```python
from build123d import *

# Parameters (mm, degrees)
SKETCH_R        = 11
PAD_DEPTH       = 15
SKETCH001_R     = 11
SKETCH001_R_2   = 5.1
POCKET_DEPTH    = 1.5
SKETCH002_R     = 11
SKETCH002_R_2   = 5.1
POCKET001_DEPTH = 10
SKETCH003_R     = 1.75
POCKET002_DEPTH = 13.501
SKETCH004_R     = 4
POCKET003_DEPTH = 15.001


with BuildPart() as part:
    # Sketch → Pad (new body)
    with BuildSketch(Plane.XY):
        Circle(SKETCH_R)
    extrude(amount=PAD_DEPTH)

    # Sketch001 (on Face3 of Pad) → Pocket (cut)
    with BuildSketch(Plane.XY.offset(15)):
        Circle(SKETCH001_R)
        Circle(SKETCH001_R_2, mode=Mode.SUBTRACT)
    extrude(amount=-POCKET_DEPTH, mode=Mode.SUBTRACT)

    # Sketch002 (on Face2 of Pocket) → Pocket001 (cut)
    with BuildSketch(Plane(origin=(0, 0, 0), x_dir=(1, 0, 0), z_dir=(0, 0, -1))):
        Circle(SKETCH002_R)
        Circle(SKETCH002_R_2, mode=Mode.SUBTRACT)
    extrude(amount=-POCKET001_DEPTH, mode=Mode.SUBTRACT)

    # Sketch003 (on Face3 of Pocket001) → Pocket002 (cut, through all)
    with BuildSketch(Plane.XY.offset(13.5)):
        with Locations((8, 0)):
            Circle(SKETCH003_R)
        with Locations((-8, 0)):
            Circle(SKETCH003_R)
        with Locations((0, 8)):
            Circle(SKETCH003_R)
        with Locations((0, -8)):
            Circle(SKETCH003_R)
    extrude(amount=-POCKET002_DEPTH, mode=Mode.SUBTRACT)

    # Sketch004 (on Face11 of Pocket002) → Pocket003 (cut, through all)
    with BuildSketch(Plane.XY.offset(15)):
        Circle(SKETCH004_R)
    extrude(amount=-POCKET003_DEPTH, mode=Mode.SUBTRACT)


solid = part.part
```
Here's how the part is built. I have some questions about the finished solid (model axes, mm). A direction names the side the tool comes from. Coordinates: 2 decimals unless noted, no trailing zeros. Loops run counter-clockwise (first coordinate to the right, second up) from the corner with the lowest first, then second, coordinate; pieces in that order, holes last. Notation, with made-up numbers: M 9,76.5 L 15,76.5 A17 cw 15,93.5 Z; hole C 7.5,-7.75 d6. An arc over 180 degrees is marked long. One line per item, written item: value.
1. Imagine slicing it at C-C (y = 0.5). List the corners of the cut face in (x, z) for me.
Geometry says:
outline: M -10.99,10 L -9.68,10 L -9.68,13.5 L -10.99,13.5 Z; M -6.32,10 L -5.08,10 L -5.08,0 L -3.97,0 L -3.97,15 L -5.08,15 L -5.08,13.5 L -6.32,13.5 Z; M 3.97,0 L 5.08,0 L 5.08,10 L 6.32,10 L 6.32,13.5 L 5.08,13.5 L 5.08,15 L 3.97,15 Z; M 9.68,10 L 10.99,10 L 10.99,13.5 L 9.68,13.5 Z
2. On a 3-axis mill with a long thin cutter (end or side, diameter ignored), from which of +Z, -Z, +X, -X, +Y, -Y can I reach the whole of each face in a straight line? I mean faces 1 (the cylindrical face through (2.4, -4.5, 14.3)), 2 (the flat face through (2, 5, 10)), 3 (the flat face through (-3, -3, 15)). Say none if no direction works.
Geometry says:
face 1: +Z
face 2: -Z
face 3: +Z, +X, -X, +Y, -Y
3. Imagine slicing it at D-D (z = 13). List the corners of the cut face in (x, y) for me.
Geometry says:
outline: C 0,0 d22; hole C -8,0 d3.5; hole C 0,0 d8; hole C 0,-8 d3.5; hole C 0,8 d3.5; hole C 8,0 d3.5
4. Imagine slicing it at B-B (x = -8). List the corners of the cut face in (y, z) for me, and give its area (3 significant figures).
Geometry says:
outline: M -7.55,10 L -1.75,10 L -1.75,13.5 L -7.55,13.5 Z; M 1.75,10 L 7.55,10 L 7.55,13.5 L 1.75,13.5 Z
area: 40.6 mm2
5. Will these pins go through, and if not, where does the flat tip stop? pin 1 Ø4.5 at (x, y) = (0, -8) entering from +Z; pin 2 Ø1.5 at (x, y) = (8, 1.5) entering from -Z; pin 3 Ø5 at (x, z) = (-4.5, 4.5) entering from +Y.
Geometry says:
pin 1: stops at z = 13.5
pin 2: stops at z = 10
pin 3: stops at y = 4.69
6. Imagine slicing it at A-A (x = 0). List the corners of the cut face in (y, z) for me, and give its area (3 significant figures).
Geometry says:
outline: M -11,10 L -9.75,10 L -9.75,13.5 L -11,13.5 Z; M -6.25,10 L -5.1,10 L -5.1,0 L -4,0 L -4,15 L -5.1,15 L -5.1,13.5 L -6.25,13.5 Z; M 4,0 L 5.1,0 L 5.1,10 L 6.25,10 L 6.25,13.5 L 5.1,13.5 L 5.1,15 L 4,15 Z; M 9.75,10 L 11,10 L 11,13.5 L 9.75,13.5 Z
area: 49.8 mm2
7. Thinking about a two-plate mould opening in X: for faces 4 (the flat face through (-3, -3, 0)), 5 (the cylindrical face through (2.4, 4.5, 4.9)), 6 (the cylindrical face through (-0.867, -3.905, 7.605)), which applies, +X half, -X half, draft (parallel to the pull), parting line (faces both ways), or undercut?
Geometry says:
face 4: draft
face 5: parting line
face 6: undercut
8. Please list where these lines run through material, in increasing order: probe 1 along Z at (x, y) = (-0.75, 5.25); probe 2 along X at (y, z) = (0.25, 14.25); probe 3 along Y at (x, z) = (-0.5, 14.25).
Geometry says:
probe 1: z = 10 to 13.5
probe 2: x = -5.09 to -3.99, 3.99 to 5.09
probe 3: y = -5.08 to -3.97, 3.97 to 5.08
